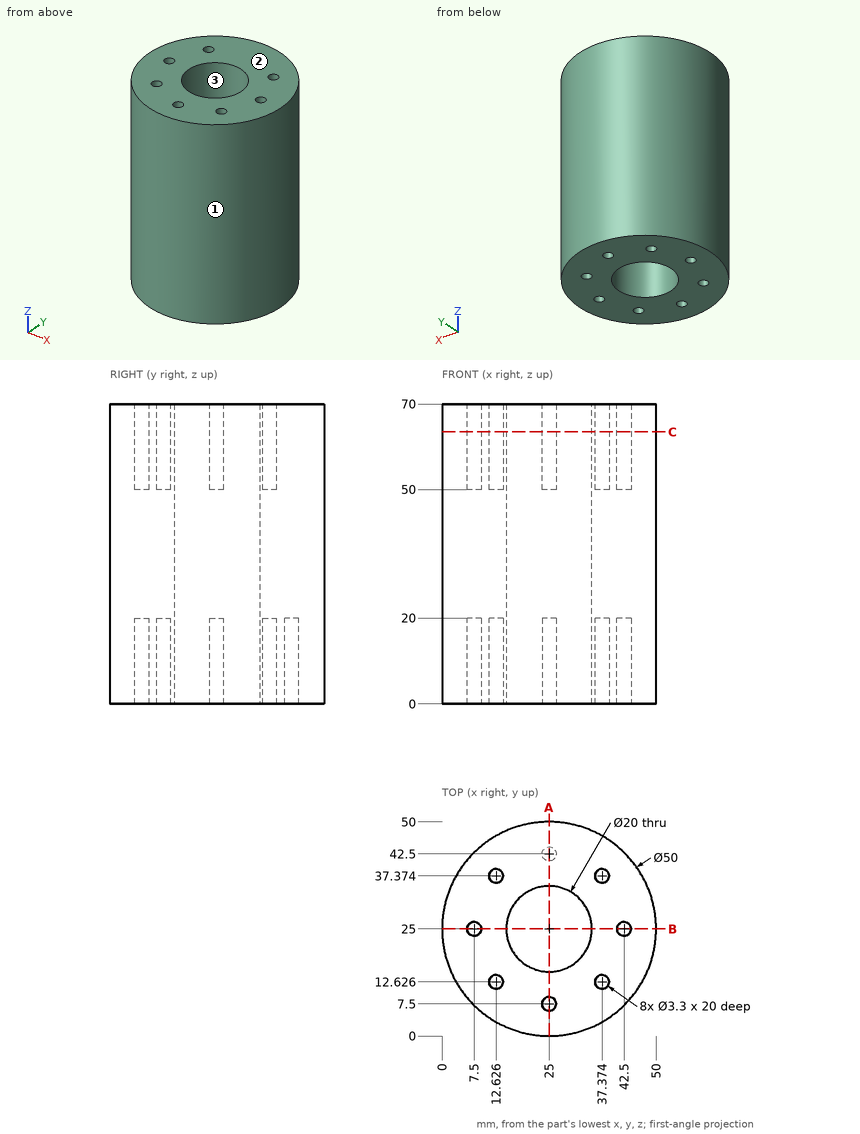
Geometry check sheet. Reference: drawing and pictorial views, mm from the part's lowest x, y, z. Give positions to 0.01 mm unless a question says otherwise; leave off trailing zeros. Order: outer loops, then holes, each group sorted by start corner. A loop starts at its lowest first (then second) coordinate and runs counter-clockwise, first axis right, second up. Notation, with made-up numbers: M 66,-14 L 81,-14 A9 cw 81,2 Z; hole C 15.5,45 d5. An arc over 180 degrees is marked long. Use one line per item in the form item = value. Start each with the question number.
Q1. Scan lines: line 1 along Y through (x, z) = (25, 59); line 2 along Y through (x, z) = (25, 14.75); line 3 along Y through (x, z) = (24, 56). Record each from-to range of solid material in increasing order. Write a range as [from, to].
Q2. Go/stop test with flat-tipped pins: pin 1 Ø4 at (x, y) = (37.37, 37.37) entering from -Z; pin 2 Ø2 at (y, z) = (32, 47) entering from +X; pin 3 Ø4 at (x, z) = (11, 38) entering from -Y; pin 4 Ø10 at (x, z) = (7.5, 28) entering from -Y. Record where each tip stops, or that it passes through.
Q3. Mould release check, pull along X, two halves, no side actions. Record for the marked faces 1, 2 and 3: +X half, -X half, draft (parallel to the pull), parting line (faces both ways), or undercut.
Q4. Section check C-C (z = 63.5). Count the separate pieces of the cut face and the enclosed holes in it, then the cut area to 3 significant figures.
Q5. Section check A-A (x = 25). Enter the section's corners in (y, z).
Q6. Section check B-B (y = 25). Enter the section's corners in (x, z).
Evaluation:
q1.line_1 = [0, 5.85], [9.15, 15], [35, 50]
q1.line_2 = [0, 5.85], [9.15, 15], [35, 40.85], [44.15, 50]
q1.line_3 = [0.02, 6.19], [8.81, 15.05], [34.95, 49.98]
q2.pin_1 = 0
q2.pin_2 = 49.27
q2.pin_3 = 3.07
q2.pin_4 = 3.35
q3.face_1 = parting line
q3.face_2 = draft
q3.face_3 = undercut
q4.separate_pieces = 1
q4.enclosed_holes = 8
q4.area = 1,590 mm2
q5.outline = M 0,0 L 5.85,0 L 5.85,20 L 9.15,20 L 9.15,0 L 15,0 L 15,70 L 9.15,70 L 9.15,50 L 5.85,50 L 5.85,70 L 0,70 Z; M 35,0 L 40.85,0 L 40.85,20 L 44.15,20 L 44.15,0 L 50,0 L 50,70 L 35,70 Z
q6.outline = M 0,0 L 5.85,0 L 5.85,20 L 9.15,20 L 9.15,0 L 15,0 L 15,70 L 9.15,70 L 9.15,50 L 5.85,50 L 5.85,70 L 0,70 Z; M 35,0 L 40.85,0 L 40.85,20 L 44.15,20 L 44.15,0 L 50,0 L 50,70 L 44.15,70 L 44.15,50 L 40.85,50 L 40.85,70 L 35,70 Z
